Work out the finished part from the listing and answer in its coordinate system (mm). Face numbers are marked on the shaded views. A direction names the side the tool comes from. Coordinates: 2 decimals unless noted, no trailing zeros. Order: outer loops, then holes, each group sorted by start corner. A loop starts at its lowest first (then second) coordinate and runs counter-clockwise, first axis right, second up.
1. Determine the mould class of the marked faces 4, 5, 6 and 7 for opening direction X: +X half, -X half, draft (parallel to the pull), parting line (faces both ways), or undercut.
2. A tool of negligible diameter and unlimited length cuts with its end or side. For the marked faces 1, 2 and 3, from which of +Z, -Z, +X, -X, +Y, -Y can it reach the whole face along a straight path? Write none if from no direction.
3. The part is cut by section C-C, the plane x = 0. Give the vertices of the cut face in (y, z), then the cut area to 3 significant figures.
4. The part is cut by section B-B, the plane y = 0. Give the vertices of the cut face in (x, z), then the cut area to 3 significant figures.
5. The part is cut by section A-A, the plane z = -185.5. Give the vertices of the cut face in (x, y), then the cut area to 3 significant figures.
6. The part is cut by section D-D, the plane z = 110. Give the vertices of the cut face in (x, y), then the cut area to 3 significant figures.
7. A flat-ended cylindrical pin translates along its axis: pin 1 Ø12 at (y, z) = (66.5, 148) entering from -X. Find the tip coordinate at first contact, or state that the pin passes through.
8. Find the intervals of material crossed by probe 1 along X at (y, z) = (24, -201); probe 2 along Z at (x, y) = (-125, 23.5); probe 3 along Z at (x, y) = (-71.5, 18.5), in increasing order.
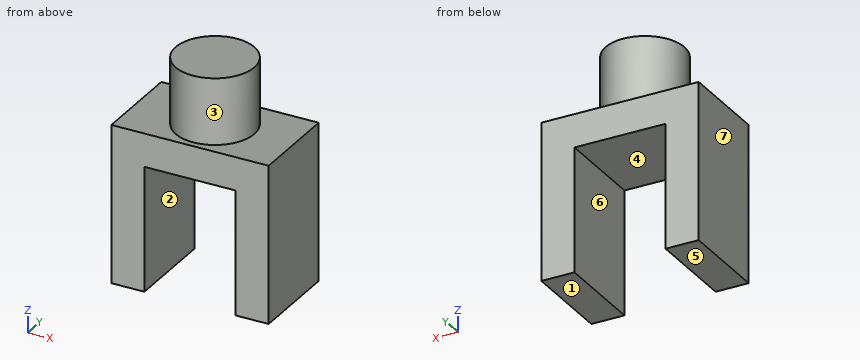
Autodesk Inventor part; units mm, degrees
ref_plane "YZ Plane" through (0, 0, 0) normal (1, 0, 0) x (0, 1, 0)
ref_plane "XZ Plane" through (0, 0, 0) normal (0, 1, 0) x (-1, 0, 0)
ref_plane "XY Plane" through (0, 0, 0) normal (0, 0, 1) x (1, 0, 0)
sketch "Sketch2" plane through (0, 0, 0) normal (0, 0, 1) x (1, 0, 0)
  line L0 (-190, 110) -> (-110, 110)
  line L1 (-110, 110) -> (-110, -110)
  line L2 (-110, -110) -> (-190, -110)
  line L3 (-190, -110) -> (-190, 110)
  line L4 (-190, 110) -> (-110, -110) construction
  line L5 (-110, 110) -> (-190, -110) construction
  line L6 (0, 0) -> (0, 15) construction
  line L7 (190, 110) -> (110, 110)
  line L8 (110, 110) -> (110, -110)
  line L9 (110, -110) -> (190, -110)
  line L10 (190, -110) -> (190, 110)
  line L11 (190, 110) -> (110, -110) construction
  line L12 (110, 110) -> (190, -110) construction
  point P0 (-150, 0)
  point P1 (-150, 0)
  point P2 (150, 0)
  point P3 (150, 0)
  dimension "d0" = 80
  dimension "d1" = 220
  dimension "d2" = 150
  dimension "d3" = 15
extrude "Extrusion1" add sketch "Sketch2" against normal blind 300
sketch "Sketch3" plane through (0, 0, 0) normal (0, 0, 1) x (1, 0, 0)
  line L0 (-190, 110) -> (-110, 110)
  line L1 (190, -110) -> (190, 110)
  line L2 (-190, 110) -> (190, 110)
  line L3 (190, 110) -> (190, -110)
  line L4 (190, -110) -> (-190, -110)
  line L5 (-190, -110) -> (-190, 110)
  point P0 (0, 0)
extrude "Extrusion2" add sketch "Sketch3" along normal blind 80
sketch "Sketch4" plane through (0, 0, 80) normal (0, 0, 1) x (1, 0, 0)
  circle A0 centre (0, 0) radius 95
  dimension "d8" = 190
extrude "Extrusion3" add sketch "Sketch4" along normal blind 160
thread "Thread1"
properties part number "09_Gripper"
Geometry says:
1. face 4: undercut
1. face 5: draft
1. face 6: undercut
1. face 7: -X half
2. face 1: -Z, +X, -X, +Y, -Y
2. face 2: -Z, +Y, -Y
2. face 3: +Z
3. outline: (-110, 0) - (110, 0) - (110, 80) - (95, 80) - (95, 240) - (-95, 240) - (-95, 80) - (-110, 80) - close
3. area: 48,000 mm2
4. outline: (-190, -300) - (-110, -300) - (-110, 0) - (110, 0) - (110, -300) - (190, -300) - (190, 80) - (95, 80) - (95, 240) - (-95, 240) - (-95, 80) - (-190, 80) - close
4. area: 109,000 mm2
5. outline: (-190, -110) - (-110, -110) - (-110, 110) - (-190, 110) - close; (110, -110) - (190, -110) - (190, 110) - (110, 110) - close
5. area: 35,200 mm2
6. outline: circle Ø190 at (0, 0)
6. area: 28,400 mm2
7. pin 1: stops at x = -73.24
8. probe 1: x = -190 to -110, 110 to 190
8. probe 2: z = -300 to 80
8. probe 3: z = 0 to 240
